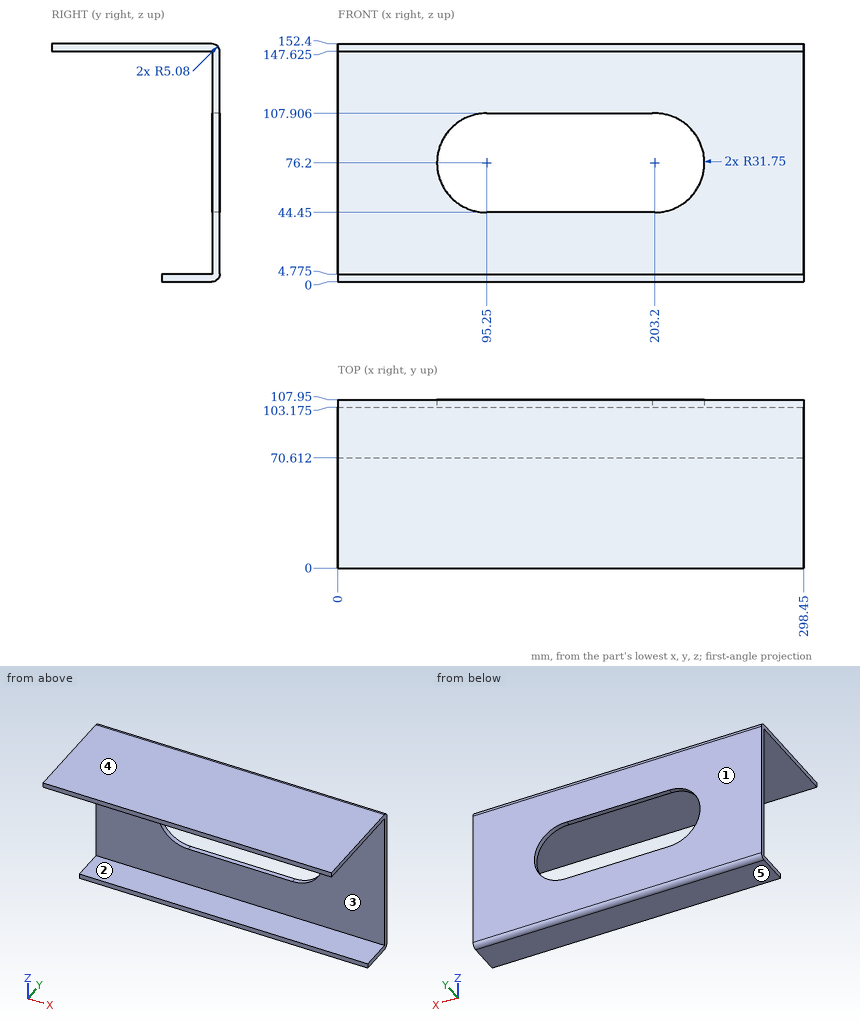
Here's the drawing with two shaded views (mm, measured from the low corner). I have some questions. A direction names the side the tool comes from. Coordinates: 2 decimals unless noted, no trailing zeros. Write item = value, one per line. Start each with the question number.
Q1. On a 3-axis mill with a long thin cutter (end or side, diameter ignored), from which of +Z, -Z, +X, -X, +Y, -Y can I reach the whole of each face in a straight line? I mean the marked faces 1 and 2. Say none if no direction works.
Q2. I'm going to push flat-ended pins straight in: pin 1 (5.5 mm diameter, centred on x = 148.5, y = 106, fed in from +Z); pin 2 (8 mm diameter, centred on x = 229.5, z = 76, fed in from -Y); pin 3 (1 mm diameter, centred on x = 163.5, y = 15.5, fed in from -Z) (3 decimals); pin 4 (5.5 mm diameter, centred on x = 120.5, z = 2.5, fed in from -Y). Where does each tip first touch, or does it pass through?
Q3. If I drill on L1, parallel to Z at x = 188.5, y = 59.5 (1 decimal); L2, parallel to Z at x = 249.5, y = 78.5 (1 decimal), over which ranges is the centre line in solid material (lowest first)? Write a range as [from, to].
Q4. Thinking about a two-plate mould opening in Z: for the marked faces 3, 4 and 5, which applies, released by +Z, released by -Z, zero draft, split by the parting line, or undercut?
Check sheet entries:
q1.face_1 = +Z, -Z, +X, -X, +Y
q1.face_2 = +X, -X, -Y
q2.pin_1 = 152.39
q2.pin_2 = through
q2.pin_3 = 147.625
q2.pin_4 = 70.61
q3.L1 = [147.6, 152.4]
q3.L2 = [0, 4.8], [147.6, 152.4]
q4.face_3 = undercut
q4.face_4 = released by +Z
q4.face_5 = released by -Z
